```python
from build123d import *

# Parameters (mm, degrees)
SKETCH2_R               = 27.873868368
BOSS_EXTRUDE1_DEPTH     = 500
CUT_EXTRUDE1_DEPTH      = 505.976972678
CUT_EXTRUDE1_DEPTH_BACK = 505.976972678
SKETCH3_W               = 228.6
SKETCH3_H               = 25.4
SKETCH3_W_2             = 68.2
SKETCH3_H_2             = 67.058155704


with BuildPart() as part:
    # Sketch2 → Boss-Extrude1 (new body)
    with BuildSketch(Plane.XY):
        Polygon((-20.337957043, 33.529077852), (-2.699269284, 33.529077852), (-2.699269284, 32.535153464), (2.699269284, 32.535153464), (2.699269284, 33.529077852), (20.337957043, 33.529077852), (20.337957043, 32.535153464), (17.271526495, 29.113021938), (27.871192843, 29.113021938), (29.262123018, 27.866666927), (29.262123018, 17.267000578), (32.013880115, 20.337957043), (33.007804503, 20.337957043), (33.007804503, 2.699269284), (32.013880115, 2.699269284), (32.013880115, -2.699269284), (33.007804503, -2.699269284), (33.007804503, -20.337957043), (32.013880115, -20.337957043), (29.262123018, -17.267000578), (29.262123018, -27.866666927), (27.871192843, -29.113021938), (17.271526495, -29.113021938), (20.337957043, -32.535153464), (20.337957043, -33.529077852), (2.699269284, -33.529077852), (2.699269284, -32.535153464), (-2.699269284, -32.535153464), (-2.699269284, -33.529077852), (-20.337957043, -33.529077852), (-20.337957043, -32.535153464), (-17.271526495, -29.113021938), (-27.871192843, -29.113021938), (-29.262123018, -27.866666927), (-29.262123018, -17.267000578), (-32.013880115, -20.337957043), (-33.007804503, -20.337957043), (-33.007804503, -2.699269284), (-32.013880115, -2.699269284), (-32.013880115, 2.699269284), (-33.007804503, 2.699269284), (-33.007804503, 20.337957043), (-32.013880115, 20.337957043), (-29.262123018, 17.267000578), (-29.262123018, 27.866666927), (-27.871192843, 29.113021938), (-17.271526495, 29.113021938), (-20.337957043, 32.535153464), align=None)
        Circle(SKETCH2_R, mode=Mode.SUBTRACT)
    extrude(amount=BOSS_EXTRUDE1_DEPTH)

    # Sketch3 → Cut-Extrude1 (cut, two sides: drawn at the far end of the back side and taken through both)
    with BuildSketch(Plane(origin=(29.262123018, 0, 0), x_dir=(0, 0, -1), z_dir=(1, 0, 0)).offset(-CUT_EXTRUDE1_DEPTH_BACK)):
        with Locations((-284.1, 20.829077852)):
            Rectangle(SKETCH3_W, SKETCH3_H)
        with Locations((-34.1, 0)):
            Rectangle(SKETCH3_W_2, SKETCH3_H_2)
    extrude(amount=CUT_EXTRUDE1_DEPTH + CUT_EXTRUDE1_DEPTH_BACK, mode=Mode.SUBTRACT)


solid = part.part
```
Here's how the part is built. I have some questions about the finished solid (model axes, mm). A direction names the side the tool comes from. Give positions to 0.01 mm unless a question says otherwise; leave off trailing zeros. Write each loop counter-clockwise with the first axis right and the second up, starting at its lowest first coordinate (ties: lowest second). Pieces come first, ordered by that corner, then holes. Notation, with made-up numbers: M 26.5,40 L 60.5,40 A20 ccw 60.5,57 Z; hole C 31.25,44.25 d5. An arc over 180 degrees is marked long. Put each result on its own line as item: value. Start each with the question number.
Item 1: If we section it at A-A, the plane x = -13: Write out the boundary of the cut face in (y, z), then the cut area to 3 significant figures.
Item 2: On a 3-axis mill with a long thin cutter (end or side, diameter ignored), from which of +Z, -Z, +X, -X, +Y, -Y can I reach the whole of each face in a straight line? I mean faces 1 (the flat face through (-12, 33.529, 118)), 2 (the flat face through (0, 29, 169.8)). Say none if no direction works.
Item 3: If we section it at B-B, the plane y = -11: Write out the boundary of the cut face in (x, z), then the cut area to 3 significant figures.
Item 4: I need wall thicknesses on L1, parallel to X at y = 0, z = 323; L2, parallel to Z at x = -21, y = 24; L3, parallel to Y at x = 18, z = 86. Which ranges of each line are inside material? Lowest first, please. Write a range as from..to.
Item 5: If we section it at D-D, the plane y = 12.5: Write out the boundary of the cut face in (x, z).
Item 6: Thinking about a two-plate mould opening in X: for faces 3 (the flat face through (-29.262, -23, 281)), 4 (the flat face through (20, -20, 500)), 5 (the flat face through (-33.008, -12, 281)), which applies, +X half, -X half, draft (parallel to the pull), parting line (faces both ways), or undercut?
Item 7: Will these pins go through, and if not, where does the flat tip stop? pin 1 (0.5 mm diameter, centred on x = 32.5, z = 340, fed in from -Y); pin 2 (1 mm diameter, centred on x = -20.5, z = 190, fed in from +Y); pin 3 (2.5 mm diameter, centred on x = 0.5, z = 140.5, fed in from +Y); pin 4 (3 mm diameter, centred on x = 10, y = 23.5, fed in from -Z).
Values:
1. outline: M -33.53,68.2 L -24.66,68.2 L -24.66,500 L -33.53,500 Z; M 24.66,68.2 L 33.53,68.2 L 33.53,169.8 L 24.66,169.8 Z; M 24.66,398.4 L 33.53,398.4 L 33.53,500 L 24.66,500 Z
1. area: 5,630 mm²
2. face 1: +Z, -Z, +X, -X, +Y
2. face 2: +X, -X, +Y
3. outline: M -33.01,68.2 L -25.61,68.2 L -25.61,500 L -33.01,500 Z; M 25.61,68.2 L 33.01,68.2 L 33.01,500 L 25.61,500 Z
3. area: 6,390 mm²
4. L1: -32.01..-27.87, 27.87..32.01
4. L2: 68.2..169.8, 398.4..500
4. L3: -33.53..-29.93, -29.11..-21.28, 21.28..29.11, 29.93..33.53
5. outline: M -33.01,68.2 L -24.91,68.2 L -24.91,169.8 L -33.01,169.8 Z; M -33.01,398.4 L -24.91,398.4 L -24.91,500 L -33.01,500 Z; M 24.91,68.2 L 33.01,68.2 L 33.01,169.8 L 24.91,169.8 Z; M 24.91,398.4 L 33.01,398.4 L 33.01,500 L 24.91,500 Z
6. face 3: undercut
6. face 4: draft
6. face 5: -X half
7. pin 1: y = -20.34
7. pin 2: y = -18.33
7. pin 3: y = 32.54
7. pin 4: through
